Part print with two shaded views. Sizes in mm from the minimum x, y, z corner. A direction names the side the tool comes from. Round coordinates to 2 decimals unless told otherwise and drop trailing zeros. Write each loop counter-clockwise with the first axis right and the second up, starting at its lowest first coordinate (ties: lowest second). Pieces come first, ordered by that corner, then holes. Notation, with made-up numbers: M 30.25,72 L 45.25,72 A20 ccw 45.25,101 Z; hole C 10,22 d2. An arc over 180 degrees is marked long. Use one line per item in the form item = value. Start each with the question number.
Item 1: Which spindle directions (+Z, -Z, +X, -X, +Y, -Y) get a long thin tool onto all of the face, cutting with end or side? Do the marked faces 1 and 2. Say none if no direction does.
Item 2: Probe L1, parallel to Y at x = 4, z = 18; L2, parallel to Z at x = 11.75, y = 25.5; L3, parallel to Z at x = 20.25, y = 63. List the from-to ranges inside material, lowest first.
Item 3: Flat gauge pins, fed straight in: pin 1 Ø3 at (x, z) = (21, 24.5) entering from +Y; pin 2 Ø7.5 at (x, y) = (11, 25) entering from +Z; pin 3 Ø3 at (x, y) = (13.5, 61.5) entering from +Z. Where does each tip first touch, or does it go through?
Item 4: Mould opens along X. For the marked faces 3, 4 and 5 say: +X half, -X half, draft (parallel to the pull), parting line (faces both ways), or undercut.
Item 5: Cut at B-B, the plane z = 68.5. Give the cut face in (x, y).
Item 6: Cut at C-C, the plane y = 13. Give the cut face in (x, z).
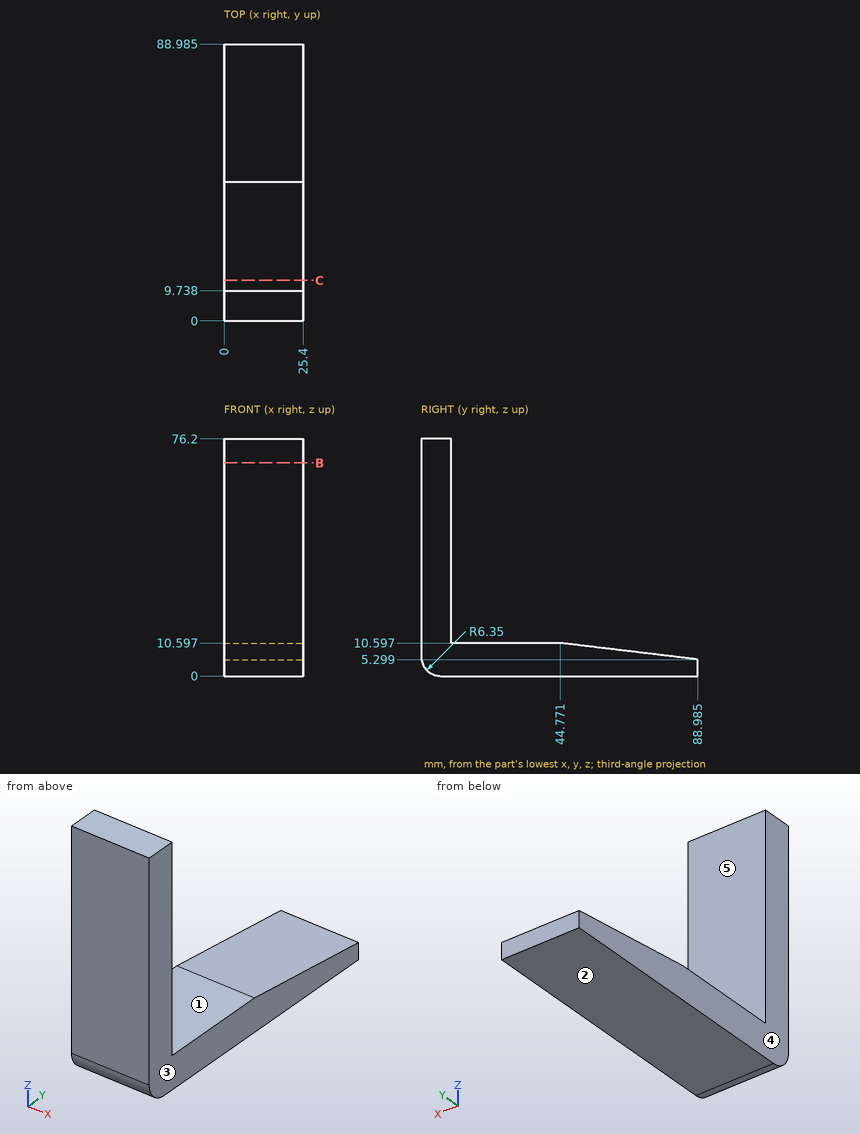
Model answer:
q1.face_1 = +Z, +X, -X, +Y
q1.face_2 = -Z, +X, -X, +Y, -Y
q2.L1 = 0 to 9.74
q2.L2 = 0 to 10.6
q2.L3 = 0 to 8.41
q3.pin_1 = 9.74
q3.pin_2 = 10.6
q3.pin_3 = 8.77
q4.face_3 = +X half
q4.face_4 = -X half
q4.face_5 = draft
q5.outline = M 0,0 L 25.4,0 L 25.4,9.74 L 0,9.74 Z
q6.outline = M 0,0 L 25.4,0 L 25.4,10.6 L 0,10.6 Z
